The drawing under review shows one solid part. Ordinate dimensions are in mm from its lowest x, y, z. Coordinates: 2 decimals unless noted, no trailing zeros. Order: outer loops, then holes, each group sorted by start corner. A loop starts at its lowest first (then second) coordinate and runs counter-clockwise, first axis right, second up.
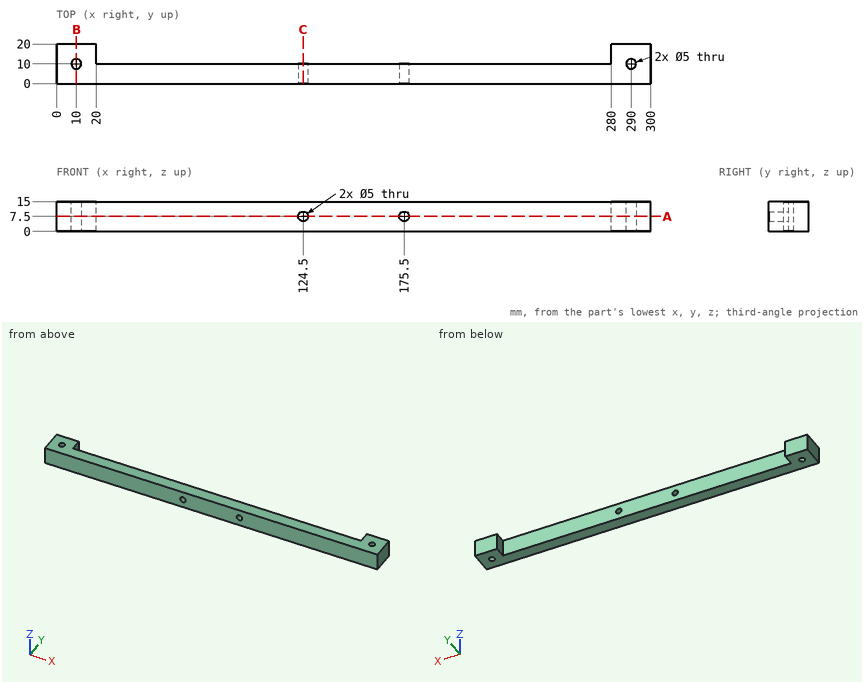
(1) We need section C-C, the plane x = 124.5. Write out the cut boundary in (y, z).
A:
outline: (0, 0) - (10, 0) - (10, 5) - (0, 5) - close; (0, 10) - (10, 10) - (10, 15) - (0, 15) - close
(2) We need section B-B, the plane x = 10. Write out the cut boundary in (y, z), and give its area (3 significant figures).
A:
outline: (0, 0) - (7.5, 0) - (7.5, 15) - (0, 15) - close; (12.5, 0) - (20, 0) - (20, 15) - (12.5, 15) - close
area: 225 mm2
(3) Wall thickness on probe 1 along X at (y, z) = (17, 9); probe 2 along X at (y, z) = (5, 6); probe 3 along Y at (x, z) = (290, 7.25): over which ranges is each line inside the solid? List them lowest first.
A:
probe 1: x = 0 to 20, 280 to 300
probe 2: x = 0 to 122.5, 126.5 to 173.5, 177.5 to 300
probe 3: y = 0 to 7.5, 12.5 to 20
(4) We need section A-A, the plane z = 7.5. Write out the cut boundary in (x, y), and give its area (3 significant figures).
A:
outline: (0, 0) - (122, 0) - (122, 10) - (20, 10) - (20, 20) - (0, 20) - close; (127, 0) - (173, 0) - (173, 10) - (127, 10) - close; (178, 0) - (300, 0) - (300, 20) - (280, 20) - (280, 10) - (178, 10) - close; hole circle Ø5 at (10, 10); hole circle Ø5 at (290, 10)
area: 3,260 mm2
(5) For pin 1 Ø4 at (x, z) = (63, 12) entering from +Y; pin 2 Ø3 at (y, z) = (14, 7.5) entering from -X, all flat-tipped, find the tip position at first contact; note any pin that passes through.
A:
pin 1: stops at y = 10
pin 2: stops at x = 0
